Geometry check sheet. Reference: the model listing, model coordinates, mm. Face numbers are marked on the shaded views. A direction names the side the tool comes from. Round coordinates to 2 decimals unless told otherwise and drop trailing zeros. Write each loop counter-clockwise with the first axis right and the second up, starting at its lowest first coordinate (ties: lowest second). Pieces come first, ordered by that corner, then holes. Notation, with made-up numbers: M -26,5.25 L 23,5.25 A22 cw 23,25.25 Z; hole C 38.5,-17 d11. An arc over 180 degrees is marked long. Use a Markdown table: item, result.
```python
from build123d import *

# Parameters (mm, degrees)
SKETCH1_W           = 53
SKETCH1_H           = 26
BOSS_EXTRUDE2_DEPTH = 4
SKETCH3_R           = 12.25
CUT_EXTRUDE2_DEPTH  = 3
CUT_EXTRUDE3_REACH  = 52.374
SKETCH4_W           = 13.5
SKETCH4_H           = 9
FILLET1_R           = 10
FILLET2_R           = 10
SKETCH5_W           = 2
SKETCH5_H           = 12
BOSS_EXTRUDE3_DEPTH = 25
SKETCH6_R           = 1.6
CUT_EXTRUDE4_DEPTH  = 64.562322282
FILLET3_R           = 10


with BuildPart() as part:
    # Sketch1 → Boss-Extrude2 (new body)
    with BuildSketch(Plane.XY):
        with Locations((19.666835682, -6.752691308)):
            Rectangle(SKETCH1_W, SKETCH1_H)
    extrude(amount=BOSS_EXTRUDE2_DEPTH)

    # Sketch3 → Cut-Extrude2 (cut)
    with BuildSketch(Plane.XY.offset(4)):
        with Locations((19.666835682, -6.752691308)):
            Circle(SKETCH3_R)
    extrude(amount=-CUT_EXTRUDE2_DEPTH, mode=Mode.SUBTRACT)

    # Sketch4 → Cut-Extrude3 (cut, up to next)
    with BuildSketch(Plane.XY.offset(4), mode=Mode.PRIVATE) as cut_extrude3_sk1:
        with Locations((-0.083164318, 1.747308692)):
            Rectangle(SKETCH4_W, SKETCH4_H)
    cut_extrude3_tool1 = extrude(cut_extrude3_sk1.sketch, amount=-CUT_EXTRUDE3_REACH, mode=Mode.PRIVATE) & part.part
    # Sketch4 → Cut-Extrude3 (cut, up to next)
    with BuildSketch(Plane.XY.offset(4), mode=Mode.PRIVATE) as cut_extrude3_sk2:
        with Locations((39.416835682, 1.747308692)):
            Rectangle(SKETCH4_W, SKETCH4_H)
    cut_extrude3_tool2 = extrude(cut_extrude3_sk2.sketch, amount=-CUT_EXTRUDE3_REACH, mode=Mode.PRIVATE) & part.part
    add(cut_extrude3_tool1.solids().sort_by_distance((-0.083164, 1.747309, 4))[0], mode=Mode.SUBTRACT)
    add(cut_extrude3_tool2.solids().sort_by_distance((39.416836, 1.747309, 4))[0], mode=Mode.SUBTRACT)

    # Fillet1
    # the kernel refuses this fillet: 10 mm, written as the material it adds along each edge
    with BuildSketch(Plane(origin=(32.666835682, -2.752691308, 4), x_dir=(0, 1, 0), z_dir=(0, 0, -1))) as fillet1_piece_1:
        with BuildLine():
            CenterArc((10, 9.949874371), FILLET1_R, 180, 84.260829523)
            Line((0, 9.949874371), (-0.2, 9.949874371))
            Line((-0.2, 9.949874371), (-0.2, 0))
            Line((-0.2, 0), (0, -0.2))
            ThreePointArc((0, -0.2), (4.5, -0.2), (8.98, -0.198997487))
            Line((8.98, -0.198997487), (9, 0))
        make_face()
    extrude(amount=4)
    with BuildSketch(Plane(origin=(6.666835682, -2.752691308, 4), x_dir=(0, 1, 0), z_dir=(0, 0, -1))) as fillet1_piece_2:
        with BuildLine():
            CenterArc((10, -9.949874371), FILLET1_R, 95.739170477, 84.260829523)
            Line((0, -9.949874371), (-0.2, -9.949874371))
            Line((-0.2, -9.949874371), (-0.2, 0))
            Line((-0.2, 0), (0, 0.2))
            ThreePointArc((0, 0.2), (4.5, 0.2), (8.98, 0.198997487))
            Line((8.98, 0.198997487), (9, 0))
        make_face()
    extrude(amount=4)

    # Fillet2
    fillet2_edges = [part.edges().sort_by_distance(p)[0] for p in [
        (6.666835682, 6.247308692, 2),
        (32.666835682, 6.247308692, 2),
    ]]
    fillet(fillet2_edges, radius=FILLET2_R)

    # Sketch5 → Boss-Extrude3 (add)
    with BuildSketch(Plane.XY.offset(4)):
        with Locations((-5.833164318, -13.752691308)):
            Rectangle(SKETCH5_W, SKETCH5_H)
        with Locations((45.166835682, -13.752691308)):
            Rectangle(SKETCH5_W, SKETCH5_H)
    extrude(amount=BOSS_EXTRUDE3_DEPTH)

    # Sketch6 → Cut-Extrude4 (cut, through all)
    with BuildSketch(Plane.ZY.offset(6.833164318)):
        with Locations(Location((23, -12.752691308, 0), (0, 0, 270))):
            Circle(SKETCH6_R)
    extrude(amount=-CUT_EXTRUDE4_DEPTH, mode=Mode.SUBTRACT)

    # Fillet3
    # the kernel refuses this fillet: 10 mm, written as the material it adds along each edge
    with BuildSketch(Plane(origin=(44.166835682, -7.752691308, 4), x_dir=(0, 1, 0), z_dir=(1, 0, 0))) as fillet3_piece_1_section:
        with BuildLine():
            CenterArc((FILLET3_R, FILLET3_R), FILLET3_R, 180, 90)
            Line((0, FILLET3_R), (0, 0))
            Line((0, 0), (FILLET3_R, 0))
        make_face()
    fillet3_piece_1 = extrude(amount=2, mode=Mode.PRIVATE)
    fillet3_piece_1 = split(fillet3_piece_1, bisect_by=Plane(origin=(45.166835682, -2.752691308, 6.440248494), z_dir=(0, -1, 0)), keep=Keep.TOP, mode=Mode.PRIVATE)
    add(fillet3_piece_1)
    with BuildSketch(Plane(origin=(-6.833164318, -7.752691308, 4), x_dir=(0, 1, 0), z_dir=(1, 0, 0))) as fillet3_piece_2_section:
        with BuildLine():
            CenterArc((FILLET3_R, FILLET3_R), FILLET3_R, 180, 90)
            Line((0, FILLET3_R), (0, 0))
            Line((0, 0), (FILLET3_R, 0))
        make_face()
    fillet3_piece_2 = extrude(amount=2, mode=Mode.PRIVATE)
    fillet3_piece_2 = split(fillet3_piece_2, bisect_by=Plane(origin=(-5.833164318, -2.752691308, 6.440248494), z_dir=(0, -1, 0)), keep=Keep.TOP, mode=Mode.PRIVATE)
    add(fillet3_piece_2)


solid = part.part
```
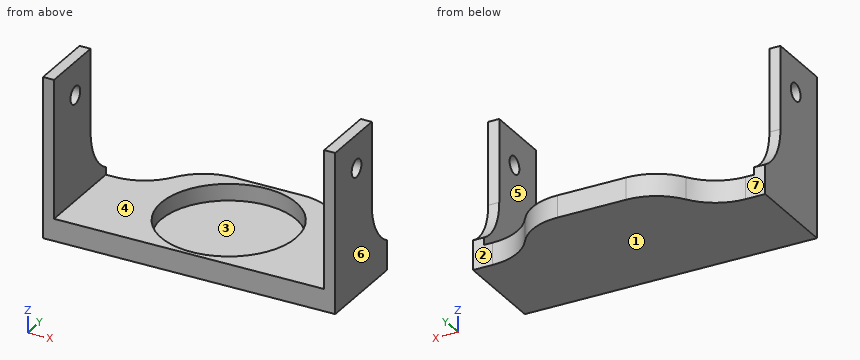
Item 1: Material ranges on line 1 along X through (y, z) = (-14.5, 13.5); line 2 along Z through (x, y) = (41, -5.75); line 3 along Z through (x, y) = (21, 2.75), recorded low to high. Write a range as from..to.
Outcome:
| item | result |
|---|---|
| line 1 | x = -6.83..-4.83, 44.17..46.17 |
| line 2 | z = 0..4 |
| line 3 | z = 0..1 |
Item 2: Cross-section at D-D, the plane y = -17.5. Record the cut outline in (x, z).
Outcome:
| item | result |
|---|---|
| outline | M -6.83,0 L 46.17,0 L 46.17,29 L 44.17,29 L 44.17,4 L 25.55,4 L 25.55,1 L 13.79,1 L 13.79,4 L -4.83,4 L -4.83,29 L -6.83,29 Z |
Item 3: Access from +Z, -Z, +X, -X, +Y, -Y to the whole of each face (thin tool, end or side, straight path). Record for the marked faces 1, 2, 3 and 4.
Outcome:
| item | result |
|---|---|
| face 1 | -Z, +X, -X, +Y, -Y |
| face 2 | +Z, -Z, +X, +Y |
| face 3 | +Z |
| face 4 | +Z, +Y, -Y |
Item 4: Mould release check, pull along X, two halves, no side actions. Record for the marked faces 5, 6 and 7: +X half, -X half, draft (parallel to the pull), parting line (faces both ways), or undercut.
Outcome:
| item | result |
|---|---|
| face 5 | undercut |
| face 6 | +X half |
| face 7 | draft |
Item 5: Cross-section at B-B, the plane z = 8.25. Record the cut outline in (x, y), and give its area (3 significant figures).
Outcome:
| item | result |
|---|---|
| outline | M -6.83,-19.75 L -4.83,-19.75 L -4.83,-5.93 L -6.83,-5.93 Z; M 44.17,-19.75 L 46.17,-19.75 L 46.17,-5.93 L 44.17,-5.93 Z |
| area | 55.3 mm2 |
Item 6: Go/stop test with flat-tipped pins: pin 1 (1.1 mm diameter, centred on x = 44, z = 1.5, fed in from +Y); pin 2 (12 mm diameter, centred on x = 37, z = 18.5, fed in from +Y); pin 3 (1 mm diameter, centred on x = -5.5, z = 24.5, fed in from +Y); pin 4 (2 mm diameter, centred on x = 13, y = -9.5, fed in from +Z). Record where each tip stops, or that it passes through.
Outcome:
| item | result |
|---|---|
| pin 1 | stops at y = -2.75 |
| pin 2 | passes through |
| pin 3 | stops at y = -7.75 |
| pin 4 | stops at z = 1 |
Item 7: Cross-section at A-A, the plane z = 23. Record the cut outline in (x, y), and give its area (3 significant figures).
Outcome:
| item | result |
|---|---|
| outline | M -6.83,-19.75 L -4.83,-19.75 L -4.83,-14.35 L -6.83,-14.35 Z; M -6.83,-11.15 L -4.83,-11.15 L -4.83,-7.75 L -6.83,-7.75 Z; M 44.17,-19.75 L 46.17,-19.75 L 46.17,-14.35 L 44.17,-14.35 Z; M 44.17,-11.15 L 46.17,-11.15 L 46.17,-7.75 L 44.17,-7.75 Z |
| area | 35.2 mm2 |
Item 8: Cross-section at C-C, the plane x = 30. Record the cut outline in (y, z), and give its area (3 significant figures).
Outcome:
| item | result |
|---|---|
| outline | M -19.75,0 L 5.37,0 L 5.37,4 L -0.17,4 L -0.17,1 L -13.33,1 L -13.33,4 L -19.75,4 Z |
| area | 61.0 mm2 |
